Model file for the job. Use its own axes, mm. A direction names the side the tool comes from. Give positions to 0.01 mm unless a question says otherwise; leave off trailing zeros. Write each loop counter-clockwise with the first axis right and the second up, starting at its lowest first coordinate (ties: lowest second). Pieces come first, ordered by that corner, then holes. Notation, with made-up numbers: (39, 59) - (82, 59) arc R26 cw to (82, 98) - close; hole circle Ø2 at (88.5, -7). An arc over 180 degrees is marked (long way). Use CSV: the item, a comma, the result in double quotes.
from build123d import *

# Parameters (mm, degrees)
F2_R            = 1
F3_DEPTH        = 3
F3_COPIES_COUNT = 8
F4_R            = 1.5
F5_DEPTH        = 0.75


# Not quite as in the source:
# - a pattern or mirror of a feature is missing from the dataset's text; its kind, count and spacing are read off the source's solid


with BuildPart() as f1:
    # F0 (on Front) → F1 (revolve)
    with BuildSketch(Plane.XZ):
        Polygon((0, 8), (0, 0), (3, 0), (3, 5), (6, 5), (6, 8), align=None)
    revolve(axis=Axis((0, 0, 4), (0, 0, -1)))

    # F2 (on face) → F3 (cut, through all)
    with BuildSketch(Plane.XY.offset(8)):
        with Locations((4.25, 0)):
            Circle(F2_R)
    f3 = extrude(amount=-F3_DEPTH, mode=Mode.SUBTRACT)

    # F3_copies: F3 ×8 about axis
    f3_copies_axis = Axis((0, 0, 0), (0, 0, 1))
    for i in range(1, F3_COPIES_COUNT):
        add(f3.rotate(f3_copies_axis, i * 360 / F3_COPIES_COUNT), mode=Mode.SUBTRACT)

    # F4 (on face) → F5 (cut)
    with BuildSketch(Plane.XY.offset(8)):
        Circle(F4_R)
    extrude(amount=-F5_DEPTH, mode=Mode.SUBTRACT)


solid = f1.part
(1) Saw through at A-A, the plane y = 0. List the corners of the cut face in (x, z), then the cut area to 4 significant figures.
Checked values:
outline,"(-6, 5) - (-5.25, 5) - (-5.25, 8) - (-6, 8) - close; (-3.25, 5) - (-3, 5) - (-3, 0) - (3, 0) - (3, 5) - (3.25, 5) - (3.25, 8) - (1.5, 8) - (1.5, 7.25) - (-1.5, 7.25) - (-1.5, 8) - (-3.25, 8) - close; (5.25, 5) - (6, 5) - (6, 8) - (5.25, 8) - close"
area,"51.75 mm^2"
(2) 3-axis set-ups, long thin cutter, end or side, ignore diameter. For faces 4 (the face through (3, 1, 5)), 5 (the face through (0, 0, 7.25)), 6 (the face through (0, 0, 0)): which of +Z, -Z, +X, -X, +Y, -Y reach the whole face in a straight line?
Checked values:
face 4,"-Z"
face 5,"+Z"
face 6,"-Z, +X, -X, +Y, -Y"
(3) Saw through at C-C, the plane x = 3.5. List the corners of the cut face in (y, z), then the cut area to 3 significant figures.
Checked values:
outline,"(-4.87, 5) - (-3.87, 5) - (-3.87, 8) - (-4.87, 8) - close; (-2.14, 5) - (-0.66, 5) - (-0.66, 8) - (-2.14, 8) - close; (0.66, 5) - (2.14, 5) - (2.14, 8) - (0.66, 8) - close; (3.87, 5) - (4.87, 5) - (4.87, 8) - (3.87, 8) - close"
area,"14.8 mm^2"
(4) Saw through at D-D, the plane z = 6. Count the separate pieces of the cut face and the enclosed holes in it, then the cut area to 3 significant figures.
Checked values:
separate pieces,"1"
enclosed holes,"8"
area,"88.0 mm^2"
(5) Pull direction Y, two halves, no side cores. Call faces 1 (the face through (-3, 0, 3)), 2 (the face through (1.2, 1.2, 8)), 3 (the face through (-1.5, 0.07, 7.63)): released by +Y, released by -Y, zero draft, split by the parting line, or undercut.
Checked values:
face 1,"split by the parting line"
face 2,"zero draft"
face 3,"undercut"
(6) Wall check: probe 1 along Y at (x, z) = (2.5, 6.5); probe 2 along Z at (x, y) = (1.5, -2.75); probe 3 along Y at (x, z) = (0, 4.25). Give the ranges that are in metal, low to high. Write a range as [from, to].
Checked values:
probe 1,"y = [-5.45, -3.87], [-2.14, 2.14], [3.87, 5.45]"
probe 2,"z = [5, 8]"
probe 3,"y = [-3, 3]"
(7) Flat gauge pins, fed straight in: P1, Ø1.5, axis at x = 4, y = -4, coming from the -Z side; P2, Ø3, axis at y = 4, z = 2, coming from the -X side. Where does each tip first touch, or does it go through?
Checked values:
P1,"stops at z = 5"
P2,"stops at x = -1.66"
